The model under review builds one solid part; all positions refer to its coordinate system, in mm. A direction names the side the tool comes from. Give positions to 0.01 mm unless a question says otherwise; leave off trailing zeros. Order: outer loops, then holes, each group sorted by start corner. A loop starts at its lowest first (then second) coordinate and runs counter-clockwise, first axis right, second up. Notation, with made-up numbers: (-10.75, 22) -> (-4.75, 22) arc R19 ccw to (-4.75, 27) -> close; hole circle Ø3 at (64.5, 63.5). An arc over 180 degrees is marked (long way). Use one line per item in the form item = value.
```python
from build123d import *

# Parameters (mm, degrees)
F0_W      = 40
F0_H      = 80
F1_DEPTH  = 8
F2_W      = 40
F2_H      = 15
F3_DEPTH  = 30
F4_W      = 40
F4_H      = 10
F5_DEPTH  = 40
F6_R      = 7.99999
F7_SIZE2  = 10
F7_SIZE   = 10
F9_DEPTH  = 5
F10_W     = 48
F10_H     = 5
F10_W_2   = 1
F11_DEPTH = 5
F12_R     = 7.5
F12_R_2   = 6
F13_DEPTH = 11
F14_R     = 2.5
F15_DEPTH = 32
F16_DEPTH = 25


# Not quite as in the source:
# - a fillet or chamfer is up to 0.001 mm smaller than in the source, because OpenCascade refuses the exact size


with BuildPart() as f1:
    # F0 (on Top) → F1 (new body)
    with BuildSketch(Plane.XY):
        with Locations((-20, 2.0996452868)):
            Rectangle(F0_W, F0_H)
    extrude(amount=F1_DEPTH)

    # F2 (on face) → F3 (join)
    with BuildSketch(Plane(origin=(0, 0, 0), x_dir=(1, 0, 0), z_dir=(0, 0, -1))):
        with Locations((-20, 5.4003547132)):
            Rectangle(F2_W, F2_H)
    extrude(amount=F3_DEPTH)

    # F4 (on face) → F5 (join)
    with BuildSketch(Plane(origin=(0, 2.0996452868, 0), x_dir=(-1, 0, 0), z_dir=(0, 1, 0))):
        with Locations((20, -25)):
            Rectangle(F4_W, F4_H)
    extrude(amount=F5_DEPTH)

    # F6 (radius 8 in the source; OpenCascade refuses exactly that, so slightly less here)
    f6_edges = [f1.edges().sort_by_distance(p)[0] for p in [
        (0, 2.099645, 8),
        (-40, 2.099645, 8),
    ]]
    fillet(f6_edges, radius=F6_R)

    # F7
    f7_edges = [f1.edges().sort_by_distance(p)[0] for p in [
        (-20, -12.900355, -30),
    ]]
    chamfer(f7_edges, length=F7_SIZE, length2=F7_SIZE2)

    # F8 (on face) → F9 (join)
    with BuildSketch(Plane.XZ.offset(37.9003547132)):
        with BuildLine():
            Line((-44, -5), (4, -5))
            ThreePointArc((4, -5), (2.8166538264, 7.2111025509), (-8, 13))
            Line((-8, 13), (-32, 13))
            ThreePointArc((-32, 13), (-42.8166538264, 7.2111025509), (-44, -5))
        make_face()
    extrude(amount=F9_DEPTH)

    # F10 (on face) → F11 (join)
    with BuildSketch(Plane(origin=(0, 0, -5), x_dir=(1, 0, 0), z_dir=(0, 0, -1))):
        with Locations((-20, 40.4003547132)):
            Rectangle(F10_W, F10_H)
        with Locations((-44.5, 40.4003547132)):
            Rectangle(F10_W_2, F10_H)
        with Locations((4.5, 40.4003547132)):
            Rectangle(F10_W_2, F10_H)
    extrude(amount=-F11_DEPTH)

    # F12 (on face) → F13 (cut)
    with BuildSketch(Plane(origin=(0, 0, -30), x_dir=(1, 0, 0), z_dir=(0, 0, -1))):
        with Locations((-20, -19.5996452868)):
            Circle(F12_R)
        with Locations((-20, -19.5996452868)):
            Circle(F12_R_2, mode=Mode.SUBTRACT)
        with Locations((-20, -19.5996452868)):
            Circle(F12_R_2)
    extrude(amount=-F13_DEPTH, mode=Mode.SUBTRACT)

    # F14 (on face) → F15 (join)
    with BuildSketch(Plane(origin=(0, 42.0996452868, 0), x_dir=(-1, 0, 0), z_dir=(0, 1, 0))):
        with Locations((20, -25)):
            Circle(F14_R)
    extrude(amount=-F15_DEPTH)

    # F12 (on face) → F16 (cut)
    with BuildSketch(Plane(origin=(0, 0, -30), x_dir=(1, 0, 0), z_dir=(0, 0, -1))):
        with Locations((-20, -19.5996452868)):
            Circle(F12_R_2)
    extrude(amount=-F16_DEPTH, mode=Mode.SUBTRACT)


solid = f1.part
```
1. For L1, parallel to Z at x = -8.5, y = 8; L2, parallel to Y at x = -39.5, z = -7; L3, parallel to Z at x = -4.5, y = 25, list the stretches that pass through material, from the lowest coordinate up.
Values:
L1 = -30 to -20, 0 to 8
L2 = -12.9 to 2.1
L3 = -30 to -20, 0 to 7.19
2. Tool access review of faces 4 (the face through (-18, 26.1, -26.5)), 5 (the face through (-20, 22, 0)), 6 (the face through (-2.281, 2.66, 5.594)): name each direction out of +Z, -Z, +X, -X, +Y, -Y from which nothing blocks a thin tool from reaching the whole face with its end or side.
Values:
face_4 = none
face_5 = +X, -X, +Y
face_6 = +Z, +X, +Y
3. Add section C-C on z = -25. Give the boundary of the cut face in (x, y).
Values:
outline = (-40, -7.9) -> (0, -7.9) -> (0, 42.1) -> (-40, 42.1) -> close; hole (-22.5, 12.53) -> (-22.5, 14.15) arc R6 ccw to (-17.5, 14.15) -> (-17.5, 12.53) arc R7.5 ccw to (-17.5, 26.67) -> (-17.5, 25.05) arc R6 ccw to (-22.5, 25.05) -> (-22.5, 26.67) arc R7.5 ccw to start
4. The part is to be moulded in two halves that separate along Z. For faces 1 (the face through (-41.091, -40.365, 9.293)), 2 (the face through (-20, -37.9, -2)), 3 (the face through (-24.2, 26.3, -20)), say which applies: +Z half, -Z half, draft (parallel to the pull), parting line (faces both ways), or undercut.
Values:
face_1 = +Z half
face_2 = draft
face_3 = undercut
5. Add section A-A on x = -20. Give the boundary of the cut face in (y, z), then the cut area to 4 significant figures.
Values:
outline = (-42.9, -5) -> (-37.9, -5) -> (-37.9, 0) -> (-12.9, 0) -> (-12.9, -20) -> (-2.9, -30) -> (12.1, -30) -> (12.1, -27.5) -> (13.6, -27.5) -> (13.6, -22.5) -> (12.1, -22.5) -> (12.1, -20) -> (2.1, -20) -> (2.1, 0) -> (42.1, 0) -> (42.1, 8) -> (-37.9, 8) -> (-37.9, 13) -> (-42.9, 13) -> close; (25.6, -27.5) -> (27.1, -27.5) -> (27.1, -30) -> (42.1, -30) -> (42.1, -20) -> (27.1, -20) -> (27.1, -22.5) -> (25.6, -22.5) -> close
area = 1,395 mm^2
6. For pin 1 Ø2.5 at (x, y) = (-30, -41.5) entering from -Z; pin 2 Ø6 at (x, z) = (-9, -19) entering from +Y; pin 3 Ø2 at (x, z) = (-11, -7) entering from -Y; pin 4 Ø10 at (x, z) = (-16.5, -12.5) entering from +Y, all flat-tipped, find the tip position at first contact; note any pin that passes through.
Values:
pin_1 = -5
pin_2 = 42.1
pin_3 = -12.9
pin_4 = 2.1
7. Add section D-D on x = -28.5. Give the boundary of the cut face in (y, z).
Values:
outline = (-42.9, -5) -> (-37.9, -5) -> (-37.9, 0) -> (-12.9, 0) -> (-12.9, -20) -> (-2.9, -30) -> (42.1, -30) -> (42.1, -20) -> (2.1, -20) -> (2.1, 0) -> (42.1, 0) -> (42.1, 8) -> (-37.9, 8) -> (-37.9, 13) -> (-42.9, 13) -> close
